```python
from build123d import *

# Parameters (mm, degrees)
SALIENTE_EXTRUIR1_DEPTH = 20
CORTAR_EXTRUIR1_DEPTH   = 5
CROQUIS4_R              = 5.371921572
CROQUIS4_R_2            = 4.964711246
CROQUIS4_R_3            = 9.020708029
CROQUIS4_W              = 29.502003405
CROQUIS4_H              = 4.3269605
SALIENTE_EXTRUIR2_DEPTH = 5
SALIENTE_EXTRUIR3_DEPTH = 7
SALIENTE_EXTRUIR4_DEPTH = 5
CROQUIS8_W              = 11.57899057
CROQUIS8_H              = 35.30452721
CROQUIS8_W_2            = 11.578990571
SALIENTE_EXTRUIR5_DEPTH = 8
CROQUIS10_W             = 11.578990571
CROQUIS10_H             = 9.157571022
CROQUIS10_W_2           = 11.57899057
SALIENTE_EXTRUIR6_DEPTH = 8


with BuildPart() as part:
    # Croquis2 → Saliente-Extruir1 (new body)
    with BuildSketch(Plane.XY):
        with BuildLine():
            Line((125.948771998, 73.831195148), (206.860426755, 73.831195148))
            ThreePointArc((206.860426755, 73.831195148), (213.931494567, 70.90226296), (216.860426755, 63.831195148))
            Line((216.860426755, 63.831195148), (216.860426755, -63.104823524))
            ThreePointArc((216.860426755, -63.104823524), (213.931494567, -70.175891336), (206.860426755, -73.104823524))
            Line((206.860426755, -73.104823524), (125.948771998, -73.104823524))
            ThreePointArc((125.948771998, -73.104823524), (118.877704186, -70.175891336), (115.948771998, -63.104823524))
            Line((115.948771998, -63.104823524), (115.948771998, 63.831195148))
            ThreePointArc((115.948771998, 63.831195148), (118.877704186, 70.90226296), (125.948771998, 73.831195148))
        make_face()
    extrude(amount=SALIENTE_EXTRUIR1_DEPTH)

    # Croquis3 → Cortar-Extruir1 (cut)
    with BuildSketch(Plane.XY.offset(20)):
        with BuildLine():
            Line((131.777213557, 1.543265948), (200.449222637, 1.543265948))
            ThreePointArc((200.449222637, 1.543265948), (203.984756543, 3.007732042), (205.449222637, 6.543265948))
            Line((205.449222637, 6.543265948), (205.449222637, 54.760552668))
            ThreePointArc((205.449222637, 54.760552668), (203.984756543, 58.296086574), (200.449222637, 59.760552668))
            Line((200.449222637, 59.760552668), (131.777213557, 59.760552668))
            ThreePointArc((131.777213557, 59.760552668), (128.241679651, 58.296086574), (126.777213557, 54.760552668))
            Line((126.777213557, 54.760552668), (126.777213557, 6.543265948))
            ThreePointArc((126.777213557, 6.543265948), (128.241679651, 3.007732042), (131.777213557, 1.543265948))
        make_face()
    extrude(amount=-CORTAR_EXTRUIR1_DEPTH, mode=Mode.SUBTRACT)

    # Croquis4 → Saliente-Extruir2 (add)
    with BuildSketch(Plane.XY.offset(20)):
        with Locations((139.552044207, -11.43761555)):
            Circle(CROQUIS4_R)
        with Locations((202.870894741, -39.254617567)):
            Circle(CROQUIS4_R_2)
        with Locations((186.137514813, -53.312706969)):
            Circle(CROQUIS4_R_3)
        with Locations((189.902130019, -11.43761555)):
            Rectangle(CROQUIS4_W, CROQUIS4_H)
        Polygon((143.285708697, -26.368371403), (148.582533347, -26.368371403), (148.582533347, -36.332523638), (158.546685582, -36.332523638), (158.546685582, -41.173023795), (148.582533347, -41.173023795), (148.582533347, -51.13717603), (143.285708697, -51.13717603), (143.285708697, -41.173023795), (133.321556462, -41.173023795), (133.321556462, -36.332523638), (143.285708697, -36.332523638), align=None)
        Polygon((177.531776564, -37.06014818), (182.312742258, -27.3361267), (187.093707951, -37.06014818), align=None)
        with BuildLine():
            Line((133.321556462, -58.731134755), (142.311995954, -58.731134755))
            ThreePointArc((142.311995954, -58.731134755), (144.543113278, -60.962252079), (142.311995954, -63.193369403))
            Line((142.311995954, -63.193369403), (133.321556462, -63.193369403))
            ThreePointArc((133.321556462, -63.193369403), (131.090439139, -60.962252079), (133.321556462, -58.731134755))
        make_face()
        with BuildLine():
            Line((152.033292864, -58.731134755), (161.913955298, -58.731134755))
            ThreePointArc((161.913955298, -58.731134755), (164.145072622, -60.962252079), (161.913955298, -63.193369403))
            Line((161.913955298, -63.193369403), (152.033292864, -63.193369403))
            ThreePointArc((152.033292864, -63.193369403), (149.802175541, -60.962252079), (152.033292864, -58.731134755))
        make_face()
    extrude(amount=SALIENTE_EXTRUIR2_DEPTH)

    # Croquis5 → Saliente-Extruir3 (add)
    with BuildSketch(Plane.XY.offset(5)):
        with BuildLine():
            Line((216.860426755, 0.363185812), (216.860426755, 8.623746765))
            ThreePointArc((216.860426755, 8.623746765), (244.254011859, -6.758756408), (252.747129342, -37.006018501))
            ThreePointArc((252.747129342, -37.006018501), (252.843911184, -40.891106139), (251.382973951, -44.492346907))
            ThreePointArc((251.382973951, -44.492346907), (251.453339476, -42.564380052), (250.139816979, -41.151345675))
            ThreePointArc((250.139816979, -41.151345675), (250.067291272, -43.138500016), (248.610877543, -44.492346907))
            ThreePointArc((248.610877543, -44.492346907), (248.688866874, -42.355493028), (247.233029791, -40.789362374))
            ThreePointArc((247.233029791, -40.789362374), (246.510434032, -43.257829455), (244.254011859, -44.492346907))
            ThreePointArc((244.254011859, -44.492346907), (245.058759657, -40.789362374), (245.273288479, -37.006018501))
            ThreePointArc((245.273288479, -37.006018501), (238.806273238, -12.436920009), (216.860426755, 0.363185812))
        make_face()
        with BuildLine():
            Line((115.948771998, 0.363185812), (115.948771998, 8.623746765))
            ThreePointArc((115.948771998, 8.623746765), (88.555186894, -6.758756408), (80.062069411, -37.006018501))
            ThreePointArc((80.062069411, -37.006018501), (79.965287568, -40.891106139), (81.426224802, -44.492346907))
            ThreePointArc((81.426224802, -44.492346907), (81.355859277, -42.564380052), (82.669381774, -41.151345675))
            ThreePointArc((82.669381774, -41.151345675), (82.741907481, -43.138500016), (84.19832121, -44.492346907))
            ThreePointArc((84.19832121, -44.492346907), (84.120331879, -42.355493028), (85.576168962, -40.789362374))
            ThreePointArc((85.576168962, -40.789362374), (86.29876472, -43.257829455), (88.555186894, -44.492346907))
            ThreePointArc((88.555186894, -44.492346907), (87.750439096, -40.789362374), (87.535910273, -37.006018501))
            ThreePointArc((87.535910273, -37.006018501), (94.002925515, -12.436920009), (115.948771998, 0.363185812))
        make_face()
    extrude(amount=SALIENTE_EXTRUIR3_DEPTH)

    # Croquis6 → Saliente-Extruir4 (add)
    with BuildSketch(Plane.XY.offset(15)):
        Polygon((170.229054201, 42.546624397), (187.733576221, 42.546624397), (194.814057039, 42.546624397), (194.814057039, 33.30266333), (187.733576221, 33.30266333), (187.733576221, 38.41634392), (170.229054201, 38.41634392), align=None)
        Polygon((137.492636039, 42.846070715), (154.99715806, 42.846070715), (162.077638877, 42.846070715), (162.077638877, 33.602109648), (154.99715806, 33.602109648), (154.99715806, 38.715790239), (137.492636039, 38.715790239), align=None)
        with BuildLine():
            ThreePointArc((147.606658689, 12.985413335), (166.370442462, 20.164117151), (184.714551358, 11.972228552))
            ThreePointArc((184.714551358, 11.972228552), (184.271283015, 10.009183036), (182.308237498, 10.452451378))
            ThreePointArc((182.308237498, 10.452451378), (166.097280974, 17.16724943), (149.88632445, 10.452451378))
            ThreePointArc((149.88632445, 10.452451378), (147.480010591, 10.579099476), (147.606658689, 12.985413335))
        make_face()
    extrude(amount=SALIENTE_EXTRUIR4_DEPTH)

    # Croquis8 → Saliente-Extruir5 (add)
    with BuildSketch(Plane.XY.offset(5)):
        with Locations((192.725958616, -90.757087129)):
            Rectangle(CROQUIS8_W, CROQUIS8_H)
        with Locations((140.083240137, -90.757087129)):
            Rectangle(CROQUIS8_W_2, CROQUIS8_H)
    extrude(amount=SALIENTE_EXTRUIR5_DEPTH)

    # Croquis10 → Saliente-Extruir6 (add)
    with BuildSketch(Plane.XY.offset(13)):
        with Locations((140.083240137, -103.830565223)):
            Rectangle(CROQUIS10_W, CROQUIS10_H)
        with Locations((192.725958616, -103.830565223)):
            Rectangle(CROQUIS10_W_2, CROQUIS10_H)
    extrude(amount=SALIENTE_EXTRUIR6_DEPTH)


solid = part.part
```
Geometry check sheet. Reference: the model listing, model coordinates, mm. A direction names the side the tool comes from. Round coordinates to 2 decimals unless told otherwise and drop trailing zeros. Loops run counter-clockwise (first coordinate to the right, second up) from the corner with the lowest first, then second, coordinate; pieces in that order, holes last. Notation, with made-up numbers: (9.25, 73) -> (57.25, 73) arc R27 cw to (57.25, 93) -> close; hole circle Ø6 at (47, 57). An arc over 180 degrees is marked (long way). Use a Markdown table: item, result.
(1) Sectioned sample at A-A (y = -24). Enter the section's corners in (x, z), then the cut area to 3 significant figures.
Calculated:
| item | result |
|---|---|
| outline | (80.59, 5) -> (88.35, 5) -> (88.35, 12) -> (80.59, 12) -> close; (115.95, 0) -> (216.86, 0) -> (216.86, 20) -> (115.95, 20) -> close; (244.46, 5) -> (252.22, 5) -> (252.22, 12) -> (244.46, 12) -> close |
| area | 2,130 mm² |
(2) Mould release check, pull along X, two halves, no side actions. Record for faces 5 (the cylindrical face through (252.854, -40.837, 8.451)), 6 (the flat face through (137.493, 41, 17)), 7 (the cylindrical face through (88.836, -6.406, 8.451)), 8 (the flat face through (140, -104, 21)): released by +X, released by -X, zero draft, split by the parting line, or undercut.
Calculated:
| item | result |
|---|---|
| face 5 | released by +X |
| face 6 | undercut |
| face 7 | released by -X |
| face 8 | zero draft |
(3) Sectioned sample at B-B (z = 2.75). Enter the section's corners in (x, y).
Calculated:
| item | result |
|---|---|
| outline | (115.95, -63.1) arc R10 ccw to (125.95, -73.1) -> (206.86, -73.1) arc R10 ccw to (216.86, -63.1) -> (216.86, 63.83) arc R10 ccw to (206.86, 73.83) -> (125.95, 73.83) arc R10 ccw to (115.95, 63.83) -> close |
(4) Go/stop test with flat-tipped pins: P1, Ø3, axis at y = 25, z = 19, coming from the +X side; P2, Ø3, axis at x = 155.5, y = 39, coming from the +Z side; P3, Ø5.5, axis at x = 147.5, z = 16.5, coming from the -Y side; P4, Ø9.5, axis at x = 194, y = -94.5, coming from the -Z side. Record where each tip stops, or that it passes through.
Calculated:
| item | result |
|---|---|
| P1 | x = 216.86 |
| P2 | z = 20 |
| P3 | y = -108.41 |
| P4 | z = 5 |
(5) Sectioned sample at D-D (x = 118.5). Enter the section's corners in (y, z), then the cut area to 3 significant figures.
Calculated:
| item | result |
|---|---|
| outline | (-69.78, 0) -> (70.5, 0) -> (70.5, 20) -> (-69.78, 20) -> close |
| area | 2,810 mm² |
(6) Sectioned sample at C-C (y = -4). Enter the section's corners in (x, z), then the cut area to 3 significant figures.
Calculated:
| item | result |
|---|---|
| outline | (90.93, 5) -> (103.46, 5) -> (103.46, 12) -> (90.93, 12) -> close; (115.95, 0) -> (216.86, 0) -> (216.86, 20) -> (115.95, 20) -> close; (229.35, 5) -> (241.88, 5) -> (241.88, 12) -> (229.35, 12) -> close |
| area | 2,190 mm² |
(7) Scan lines: probe 1 along Y at (x, z) = (190.5, 16.5); probe 2 along X at (y, z) = (13, 16.25); probe 3 along X at (y, z) = (-75, 9.25). Record each from-to range of solid material in increasing order.
Calculated:
| item | result |
|---|---|
| probe 1 | -108.41 to -99.25, -73.1 to 1.54, 33.3 to 42.55, 59.76 to 73.83 |
| probe 2 | 115.95 to 126.78, 147.62 to 152.92, 179.28 to 183.69, 205.45 to 216.86 |
| probe 3 | 134.29 to 145.87, 186.94 to 198.52 |
(8) Set-up check for faces 1 (the flat face through (157, -63.193, 22)), 2 (the flat face through (186.936, -95, 11)), 3 (the flat face through (153, 39, 20)), 4 (the cylindrical face through (128.281, 58.335, 17.535)): record each of +Z, -Z, +X, -X, +Y, -Y from which the full face is reachable in a straight line by a thin tool's end or side.
Calculated:
| item | result |
|---|---|
| face 1 | +Z, +X, -X, -Y |
| face 2 | +Z, -Z, -Y |
| face 3 | +Z, +X, -X, +Y |
| face 4 | +Z |
